Work out the finished part from the listing and answer in its coordinate system (mm). Face numbers are marked on the shaded views. A direction names the side the tool comes from. Round coordinates to 2 decimals unless told otherwise and drop trailing zeros. Loops run counter-clockwise (first coordinate to the right, second up) from the corner with the lowest first, then second, coordinate; pieces in that order, holes last. Notation, with made-up numbers: M 19.25,-7 L 70.25,-7 A7 cw 70.25,5 Z; hole C 5.25,-36 d6. An arc over 180 degrees is marked long. One line per item, written item: value.
```python
from build123d import *

# Parameters (mm, degrees)
FILLET1_R          = 0.1
CUT_EXTRUDE1_DEPTH = 2


with BuildPart() as part:
    # Sketch1 → Revolve1 (revolve)
    with BuildSketch(Plane.XY, mode=Mode.PRIVATE) as revolve1_sk:
        Polygon((-0.8, 0), (-0.8, 2), (-0.222649731, 3), (0, 3), (0, 1.345), (0.9, 1.345), (1.4, 1.5), (5, 1.5), (5, 0), align=None)
    revolve(revolve1_sk.sketch.rotate(Axis((-0.8, 0, 0), (1, 0, 0)), 180), axis=Axis((-0.8, 0, 0), (1, 0, 0)))

    # Fillet1
    fillet1_edges = [part.edges().sort_by_distance(p)[0] for p in [
        (0, 1.345, 0),
    ]]
    fillet(fillet1_edges, radius=FILLET1_R)

    # Sketch2 → Cut-Extrude1 (cut)
    with BuildSketch(Plane.ZY.offset(0.8)):
        Polygon((0, 0.866025404), (-0.75, 0.433012702), (-0.75, -0.433012702), (0, -0.866025404), (0.75, -0.433012702), (0.75, 0.433012702), align=None)
    extrude(amount=-CUT_EXTRUDE1_DEPTH, mode=Mode.SUBTRACT)

    # Sketch3 → Cut-Revolve1 (revolve, cut)
    with BuildSketch(Plane.XY, mode=Mode.PRIVATE) as cut_revolve1_sk:
        Polygon((1.2, 0), (1.2, 0.75), (1.650645464, 0), align=None)
    revolve(cut_revolve1_sk.sketch.rotate(Axis((1.2, 0, 0), (1, 0, 0)), 180), axis=Axis((1.2, 0, 0), (1, 0, 0)), mode=Mode.SUBTRACT)


solid = part.part
```
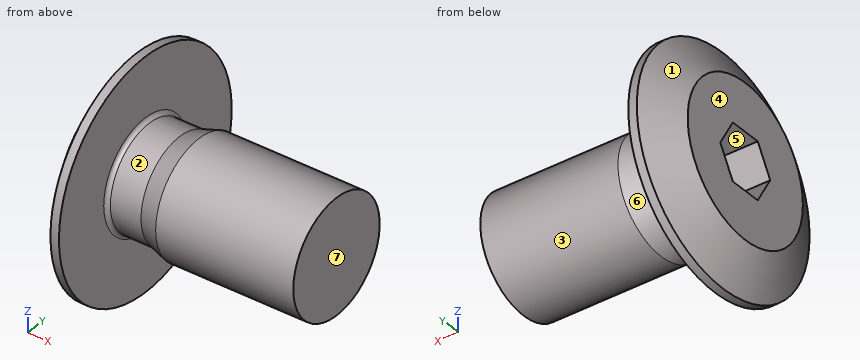
1) Each of these flat-tipped pins is pushed along its axis until it touches: pin 1 (1.5 mm diameter, centred on x = 0.5, z = -1.5, fed in from +Y); pin 2 (1 mm diameter, centred on x = 2.5, y = -0.5, fed in from +Z). Where does it stop, or does it pass through?
Check values:
pin 1: y = 2.85
pin 2: z = 1.5
2) For the marked faces 1, 2 and 3, determine the directions among +Z, -Z, +X, -X, +Y, -Y from which every point of the face is accessible in a straight line to the end or side of a thin tool.
Check values:
face 1: -X
face 2: none
face 3: +X
3) Find section B-B (x = 1.55). Give the vertices of the cut face in (y, z) (1 decimal), then the cut area to 3 significant figures.
Check values:
outline: C 0,0 d3; hole C 0,0 d0.3
area: 6.98 mm2
4) Find the intervals of material crossed by probe 1 along X at (y, z) = (0.35, -1.6); probe 2 along X at (y, z) = (2.6, -0.4); probe 3 along Y at (x, z) = (2.4, -0.8), in increasing order. Write a range as from..to.
Check values:
probe 1: -0.8..0
probe 2: -0.44..0
probe 3: -1.27..1.27
5) The mould has two halves that part along X. Classify the marked faces 4, 5, 6 and 7: +X half, -X half, draft (parallel to the pull), parting line (faces both ways), or undercut.
Check values:
face 4: -X half
face 5: draft
face 6: undercut
face 7: +X half
6) Find section A-A (x = 2.4). Give the vertices of the cut face in (y, z), then the cut area to 3 significant figures.
Check values:
outline: C 0,0 d3
area: 7.07 mm2
